Could you check a few things on this model? Use its own coordinates, in mm. A direction names the side the tool comes from. Give positions to 0.01 mm unless a question says otherwise; leave off trailing zeros. Write each loop counter-clockwise with the first axis right and the second up, starting at its lowest first coordinate (ties: lowest second). Pieces come first, ordered by that corner, then holes. Notation, with made-up numbers: (62, 70.25) - (121, 70.25) arc R24 ccw to (121, 85.25) - close; hole circle Ø11 at (-17, -34.5). An arc over 180 degrees is marked (long way). Answer as a JSON object with one key per item and string values. Group by question number.
```python
from build123d import *

# Parameters (mm, degrees)
F1_DEPTH = 25


with BuildPart() as f1:
    # F0 (on Front) → F1 (new body)
    with BuildSketch(Plane.XZ):
        with BuildLine():
            Line((-35.470672, 3.699372), (-49.148146, -47.345653))
            ThreePointArc((-49.148146, -47.345653), (-46.772589, -66.102477), (-31.944444, -77.832263))
            ThreePointArc((-31.944444, -77.832263), (0, -82.358046), (31.944444, -77.832263))
            ThreePointArc((31.944444, -77.832263), (46.772589, -66.102477), (49.148146, -47.345653))
            Line((49.148146, -47.345653), (35.522421, 3.506244))
            ThreePointArc((35.522421, 3.506244), (35.496354, 3.602756), (35.470672, 3.699372))
            ThreePointArc((35.470672, 3.699372), (35.788024, 17.547763), (43.429453, 29.101429))
            ThreePointArc((43.429453, 29.101429), (43.688987, 29.324619), (43.946501, 29.550138))
            ThreePointArc((43.946501, 29.550138), (38.94623, 50.174676), (24.731334, 34.416789))
            ThreePointArc((24.731334, 34.416789), (25.119215, 33.645622), (25.439145, 32.843876))
            ThreePointArc((25.439145, 32.843876), (17.674598, 19.683186), (6, 29.541975))
            Line((6, 29.541975), (6, 143.131175))
            ThreePointArc((6, 143.131175), (7.314658, 147.525057), (10.826549, 150.474826))
            ThreePointArc((10.826549, 150.474826), (16.266553, 155.169201), (18.049311, 162.12999))
            ThreePointArc((18.049311, 162.12999), (19.193699, 167.920002), (22.959953, 172.464142))
            ThreePointArc((22.959953, 172.464142), (23.717633, 188.010173), (8.362425, 185.466407))
            Line((8.362425, 185.466407), (-8.611184, 155.4601))
            ThreePointArc((-8.611184, 155.4601), (-8.591447, 152.471612), (-6, 150.983036))
            Line((-6, 150.983036), (-6, 51.53346))
            ThreePointArc((-6, 51.53346), (-8.985735, 45.29991), (-15.714286, 43.719292))
            ThreePointArc((-15.714286, 43.719292), (-36.351172, 35.70078), (-36.950613, 13.568941))
            ThreePointArc((-36.950613, 13.568941), (-35.18295, 8.788259), (-35.470672, 3.699372))
        make_face()
        with BuildLine():
            ThreePointArc((35.470672, 3.699372), (35.496354, 3.602756), (35.522421, 3.506244))
            Line((35.522421, 3.506244), (35.470672, 3.699372))
        make_face()
        with BuildLine():
            ThreePointArc((25.439145, 32.843876), (25.119215, 33.645622), (24.731334, 34.416789))
            ThreePointArc((24.731334, 34.416789), (25.056942, 33.617599), (25.439145, 32.843876))
        make_face()
    extrude(amount=F1_DEPTH)


solid = f1.part
```
(1) I want a section at C-C, the plane x = -24. Please give me the cut outline in (y, z).
(2) I need wall thicknesses on L1, parallel to X at y = -1, z = -47.5; L2, parallel to X at y = -1, z = 89.5; L3, parallel to Z at x = 16, y = -15.75. Which ranges of each line are inside material? Lowest first, please.
(3) Will these pins go through, and if not, where does the flat tip stop? P1, Ø7.5, axis at y = -14.5, z = 63.5, coming from the +X side; P2, Ø1.5, axis at x = -29.5, y = -13, coming from the -Z side; P3, Ø12, axis at x = -29, y = -3, coming from the +Z side.
(4) If we mould it in two halves opening along Z, with no side actions, what happens to faces 1 (the flat face through (-1, -25, -5)), 2 (the flat face through (-0.006, -12.325, 170.673)), 3 (the flat face through (-42.214, -12.325, -21.466)), 4 (the cylindrical face through (-0.453, -12.325, -82.357))? For each: +Z half, -Z half, draft (parallel to the pull), parting line (faces both ways), or undercut.
(5) I want a section at A-A, the plane y = -12.5. Please give me the cut outline in (x, z), and give its area (3 significant figures).
(6) For faces 5 (the flat face through (-6, -12, 102)), 6 (the flat face through (-1, 0, -5)), 7 (the cylindrical face through (7.3, -12.3, 147.5)), 8 (the flat face through (6, -12, 86)), which set-ups out of +Z, -Z, +X, -X, +Y, -Y let a thin tool reach every point of the face, with its end or its side?
(7) I want a section at B-B, the plane z = 8. Please give me the cut outline in (x, y), and give its area (3 significant figures).
Entries:
{
 "1": {"outline": "(-25, -79.83) - (0, -79.83) - (0, 43.78) - (-25, 43.78) - close"},
 "2": {"L1": "-49.19 to 49.19", "L2": "-6 to 6", "L3": "-81.24 to 19.54, 154.76 to 190.49"},
 "3": {"P1": "x = 6", "P2": "z = -78.71", "P3": "z = 43.96"},
 "4": {"face 1": "draft", "face 2": "+Z half", "face 3": "undercut", "face 4": "-Z half"},
 "5": {"outline": "(-49.15, -47.35) arc R25 ccw to (-31.94, -77.83) arc R115 ccw to (31.94, -77.83) arc R25 ccw to (49.15, -47.35) - (35.52, 3.51) - (35.47, 3.7) arc R25 cw to (43.43, 29.1) arc R38.01 ccw to (43.95, 29.55) arc R12 ccw (long way) to (24.73, 34.42) arc R12 ccw to (25.44, 32.84) arc R10 cw (long way) to (6, 29.54) - (6, 143.13) arc R8 cw to (10.83, 150.47) arc R12 ccw to (18.05, 162.13) arc R12 cw to (22.96, 172.46) arc R10 ccw (long way) to (8.36, 185.47) - (-8.61, 155.46) arc R3 ccw to (-6, 150.98) - (-6, 51.53) arc R8 cw to (-15.71, 43.72) arc R20 ccw to (-36.95, 13.57) arc R12.5 cw to (-35.47, 3.7) - close", "area": "12,200 mm^2"},
 "6": {"face 5": "-X, +Y, -Y", "face 6": "+Z, -Z, +X, -X, +Y", "face 7": "+X, +Y, -Y", "face 8": "+Y, -Y"},
 "7": {"outline": "(-35.09, -25) - (34.73, -25) - (34.73, 0) - (-35.09, 0) - close", "area": "1,750 mm^2"}
}
